```python
from build123d import *

# Parameters (mm, degrees)
CYLINDER103_R          = 7
CYLINDER103_DEPTH      = 9
CYLINDER104_W          = 9
CYLINDER104_H          = 9
CYLINDER104_ANGLE      = 236
CUT006_ROLL_ANGLE      = -90
CUT006_PITCH_ANGLE     = -30
CUT006_PLACEMENT_ANGLE = -90


with BuildPart() as syringe_hole:
    # Cylinder103 → Cylinder103 (new body)
    with BuildSketch(Plane.XY):
        Circle(CYLINDER103_R)
    extrude(amount=CYLINDER103_DEPTH)


with BuildPart() as syringe_hole_cut:
    # Cylinder104 → Cylinder104 (revolve)
    with BuildSketch(Plane.XZ):
        with Locations((4.5, 4.5)):
            Rectangle(CYLINDER104_W, CYLINDER104_H)
    revolve(axis=Axis((0, 0, 0), (0, 0, 1)), revolution_arc=CYLINDER104_ANGLE)

    # Cut006: cut syringe hole
    add(syringe_hole.part, mode=Mode.SUBTRACT)


with BuildPart() as syringe_hole_cut_1:
    # Cut006 roll: moved
    add(syringe_hole_cut.part.rotate(Axis((0, 0, 0), (1, 0, 0)), CUT006_ROLL_ANGLE))


with BuildPart() as syringe_hole_cut_2:
    # Cut006 pitch: moved
    add(syringe_hole_cut_1.part.rotate(Axis((0, 0, 0), (0, 1, 0)), CUT006_PITCH_ANGLE))


with BuildPart() as syringe_hole_cut_3:
    # Cut006 placement: moved
    add(syringe_hole_cut_2.part.moved(Location((111, 26, 21.5))).rotate(Axis((111, 26, 21.5), (0, 0, 1)), CUT006_PLACEMENT_ANGLE))


solid = syringe_hole_cut_3.part
```
Model file for the job. Use its own axes, mm. A direction names the side the tool comes from. Give positions to 0.01 mm unless a question says otherwise; leave off trailing zeros. Order: outer loops, then holes, each group sorted by start corner. A loop starts at its lowest first (then second) coordinate and runs counter-clockwise, first axis right, second up.
1) Wall check: probe 1 along Y at (x, z) = (116.5, 21.5); probe 2 along Z at (x, y) = (115.5, 26); probe 3 along Z at (x, y) = (113, 21.75). Give the ranges that are in metal, low to high.
2) Saw through at A-A, the plane z = 21.5. Write the cut outline in (x, y), then the cut area to 3 significant figures.
3) Saw through at B-B, the plane y = 32.75. Write the cut outline in (x, z).
4) Mould opens along Z. For faces 3 (the flat face through (111, 25, 14)), 4 (the cylindrical face through (115.437, 25.554, 14.514)), 5 (the flat face through (115.563, 19.084, 25.493)) say: +Z half, -Z half, draft (parallel to the pull), parting line (faces both ways), or undercut.
5) Saw through at C-C, the plane x = 114. Write the cut outline in (y, z), then the cut area to 3 significant figures.
6) 3-axis set-ups, long thin cutter, end or side, ignore diameter. For faces 1 (the cylindrical face through (115.56, 25.43, 12.52)), 2 (the flat face through (115.56, 33.18, 25)): which of +Z, -Z, +X, -X, +Y, -Y reach the whole face in a straight line?
7) Saw through at D-D, the plane y = 26. Write the cut outline in (x, z), then the cut area to 3 significant figures.
8) Pin check, flat tips, straight feed: pin 1 (3 mm diameter, centred on x = 114.5, y = 28.5, fed in from +Z); pin 2 (4 mm diameter, centred on x = 112, y = 31.5, fed in from -Z); pin 3 (1.5 mm diameter, centred on x = 118.5, z = 14, fed in from -Y). Stop position of each tip, or through.
Computed:
1. probe 1: y = 17 to 19, 33 to 35
1. probe 2: z = 12.5 to 14.5
1. probe 3: z = 13.57 to 15.94
2. outline: (111, 17) - (120, 17) - (120, 19) - (111, 19) - close; (111, 33) - (120, 33) - (120, 35) - (111, 35) - close
2. area: 36.0 mm2
3. outline: (111, 15.55) - (120, 15.55) - (120, 19.65) - (111, 19.65) - close; (111, 23.35) - (120, 23.35) - (120, 24.79) - (111, 24.79) - close
4. face 3: draft
4. face 4: undercut
4. face 5: +Z half
5. outline: (18.21, 26) arc R9 ccw (long way) to (34.09, 25.45) - (32.29, 24.57) arc R7 cw (long way) to (19.94, 25) - close
5. area: 65.9 mm2
6. face 1: +X, -X
6. face 2: +Z, +X, -X
7. outline: (111, 12.5) - (120, 12.5) - (120, 14.5) - (111, 14.5) - close
7. area: 18.0 mm2
8. pin 1: stops at z = 15.76
8. pin 2: stops at z = 13.21
8. pin 3: stops at y = 20.05
